Here's how the part is built. I have some questions about the finished solid (model axes, mm). A direction names the side the tool comes from. Coordinates: 2 decimals unless noted, no trailing zeros. Write each loop counter-clockwise with the first axis right and the second up, starting at its lowest first coordinate (ties: lowest second). Pieces come first, ordered by that corner, then holes. Notation, with made-up numbers: (59.5, -16.75) - (104.5, -16.75) arc R23 ccw to (104.5, 22.25) - close; hole circle Ø8 at (2.5, 77). An arc over 180 degrees is marked (long way). Answer in a Markdown table with one row per item. Add a question column.
Item 1: Which directions (+Z, -Z, +X, -X, +Y, -Y) give clear straight access to the entire face, cutting with the end or side of a thin tool? Please do faces 5 (the face through (-26.06, 16.22, -24.2)), 6 (the face through (20.871, 16.216, -9.547)).
Item 2: Imagine slicing it at B-B (x = 7.5). Please give me the cut outline in (y, z).
Item 3: We'd pull the mould along Z, two halves only. Please class faces 1 (the face through (-35, 0, -49)), 2 (the face through (-28.89, 16.22, -22.76)), 3 (the face through (30.873, 16.216, -35.379)), 4 (the face through (30.3, 16.2, -94.4)): +Z half, -Z half, draft (parallel to the pull), parting line (faces both ways), or undercut.
Item 4: Imagine slicing it at A-A (z = -50). Please give me the cut outline in (x, y).
Item 5: I'm going to push flat-ended pins straight in: pin 1 (4 mm diameter, centred on x = 9, y = 11, fed in from -Z); pin 2 (4 mm diameter, centred on x = -16.5, y = 27, fed in from -Z); pin 3 (10 mm diameter, centred on x = -13, y = 24, fed in from +Z). Where does each tip first touch, or does it pass through?
Item 6: If I drill on probe 1 along Z at (x, y) = (-23, 24.5); probe 2 along Z at (x, y) = (9, 24); probe 3 along X at (y, z) = (16.5, -76), over which ranges is the centre line in solid material (lowest first)? Write a range as from..to.
from build123d import *

# Parameters (mm, degrees)
EXTRUDE_THIN1_DEPTH = 32.893


with BuildPart() as part:
    # Sketch1 → Extrude-Thin1 (new body)
    with BuildSketch(Plane(origin=(0, 0, 0), x_dir=(1, 0, 0), z_dir=(0, 1, 0))):
        with BuildLine():
            ThreePointArc((16.859690416, 4.188302755), (20.925357953, 9.624263697), (24.673792776, 15.283641778))
            ThreePointArc((24.673792776, 15.283641778), (28.835872744, 22.655056116), (32.358402849, 30.352616811))
            ThreePointArc((32.358402849, 30.352616811), (33.886605852, 34.379502928), (35.21947344, 38.475193372))
            ThreePointArc((35.21947344, 38.475193372), (37.058530457, 45.779269739), (38.249723875, 53.216521954))
            ThreePointArc((38.249723875, 53.216521954), (38.73447294, 59.406515206), (38.763430781, 65.615392687))
            ThreePointArc((38.763430781, 65.615392687), (37.788410014, 79.600485429), (34.645449796, 93.262669938))
            ThreePointArc((34.645449796, 93.262669938), (32.487336087, 96.704142568), (28.913228351, 98.634671649))
            ThreePointArc((28.913228351, 98.634671649), (14.556820296, 101.307748109), (0, 102.469975666))
            ThreePointArc((0, 102.469975666), (-14.556820296, 101.307748109), (-28.913228351, 98.634671649))
            ThreePointArc((-28.913228351, 98.634671649), (-32.487336087, 96.704142568), (-34.645449796, 93.262669938))
            ThreePointArc((-34.645449796, 93.262669938), (-37.788410014, 79.600485429), (-38.763430781, 65.615392687))
            ThreePointArc((-38.763430781, 65.615392687), (-38.73447294, 59.406515206), (-38.249723875, 53.216521954))
            ThreePointArc((-38.249723875, 53.216521954), (-37.058530457, 45.779269739), (-35.21947344, 38.475193372))
            ThreePointArc((-35.21947344, 38.475193372), (-33.886605846, 34.37950291), (-32.358402835, 30.352616775))
            ThreePointArc((-32.358402835, 30.352616775), (-28.835872735, 22.655056099), (-24.673792776, 15.283641778))
            ThreePointArc((-24.673792776, 15.283641778), (-20.925357849, 9.62426355), (-16.859690192, 4.188302473))
            ThreePointArc((-16.859690192, 4.188302473), (-9.362082274, -1.817051595), (0, -3.968752666))
            ThreePointArc((0, -3.968752666), (9.362082435, -1.817051517), (16.859690416, 4.188302755))
        make_face()
        with BuildLine():
            ThreePointArc((14.372541639, 6.161806229), (18.329513357, 11.452436511), (21.9777336, 16.960510859))
            ThreePointArc((21.9777336, 16.960510859), (26.007427238, 24.097457247), (29.417913618, 31.550176027))
            ThreePointArc((29.417913618, 31.550176027), (30.891950162, 35.434331017), (32.177574869, 39.384851595))
            ThreePointArc((32.177574869, 39.384851595), (33.948557442, 46.418560629), (35.095657703, 53.580515883))
            ThreePointArc((35.095657703, 53.580515883), (35.563525818, 59.570235573), (35.587965764, 65.578150788))
            ThreePointArc((35.587965764, 65.578150788), (34.652553918, 79.102488225), (31.615324304, 92.314525718))
            ThreePointArc((31.615324304, 92.314525718), (30.317885926, 94.385927862), (28.167840685, 95.548407388))
            ThreePointArc((28.167840685, 95.548407388), (14.1814691, 98.154719953), (0, 99.29375))
            ThreePointArc((0, 99.29375), (-14.1814691, 98.154719953), (-28.167840685, 95.548407388))
            ThreePointArc((-28.167840685, 95.548407388), (-30.317885926, 94.385927862), (-31.615324304, 92.314525718))
            ThreePointArc((-31.615324304, 92.314525718), (-34.652553918, 79.102488225), (-35.587965764, 65.578150788))
            ThreePointArc((-35.587965764, 65.578150788), (-35.563525818, 59.570235573), (-35.095657703, 53.580515883))
            ThreePointArc((-35.095657703, 53.580515883), (-33.948557442, 46.418560629), (-32.177574869, 39.384851595))
            ThreePointArc((-32.177574869, 39.384851595), (-30.891950162, 35.434331017), (-29.417913618, 31.550176027))
            ThreePointArc((-29.417913618, 31.550176027), (-26.007427238, 24.097457247), (-21.9777336, 16.960510859))
            ThreePointArc((-21.9777336, 16.960510859), (-18.329513357, 11.452436511), (-14.372541639, 6.161806229))
            ThreePointArc((-14.372541639, 6.161806229), (-7.981004402, 1.041838599), (0, -0.79375))
            ThreePointArc((0, -0.79375), (7.981004402, 1.041838599), (14.372541639, 6.161806229))
        make_face(mode=Mode.SUBTRACT)
    extrude(amount=EXTRUDE_THIN1_DEPTH)


solid = part.part
Here are the results:
| question | item | result |
|---|---|---|
| 1 | face 5 | +Y, -Y |
| 1 | face 6 | +Z, +X, +Y, -Y |
| 2 | outline | (0, -102.06) - (32.89, -102.06) - (32.89, -98.88) - (0, -98.88) - close; (0, -0.82) - (32.89, -0.82) - (32.89, 2.61) - (0, 2.61) - close |
| 3 | face 1 | draft |
| 3 | face 2 | +Z half |
| 3 | face 3 | undercut |
| 3 | face 4 | undercut |
| 4 | outline | (-37.82, 0) - (-34.6, 0) - (-34.6, 32.89) - (-37.82, 32.89) - close; (34.6, 0) - (37.82, 0) - (37.82, 32.89) - (34.6, 32.89) - close |
| 5 | pin 1 | stops at z = -102.1 |
| 5 | pin 2 | stops at z = -101.32 |
| 5 | pin 3 | stops at z = 2.42 |
| 6 | probe 1 | z = -99.92..-96.69, -18.64..-12.67 |
| 6 | probe 2 | z = -101.93..-98.74, -1.57..1.99 |
| 6 | probe 3 | x = -38.25..-35.06, 35.06..38.25 |
